Check sheet for the modelled part. Datum: model origin and axes. Units: mm. Face numbers are marked on the shaded views. A direction names the side the tool comes from. Give positions to 0.01 mm unless a question says otherwise; leave off trailing zeros. Order: outer loops, then holes, each group sorted by start corner. A loop starts at its lowest first (then second) coordinate and runs counter-clockwise, first axis right, second up. Notation, with made-up numbers: (47, 78.5) -> (83, 78.5) arc R14 ccw to (83, 87.5) -> close; hole circle Ø8 at (78.5, -37.75). An arc over 180 degrees is marked (long way). Answer in a Markdown table with one row per item. Add a question column.
(1) Set-up check for the marked faces 4, 5 and 6: record each of +Z, -Z, +X, -X, +Y, -Y from which the full face is reachable in a straight line by a thin tool's end or side.
(2) Cross-section at B-B (x = -26). Record the cut outline in (y, z).
(3) Thickness scan on L1, parallel to Z at x = -17.5, y = 36.5; L2, parallel to Y at x = -31, z = 6.5; L3, parallel to Z at x = -26.5, y = 9. Record the ranges inside material, lowest first. Write a range as [from, to].
(4) Go/stop test with flat-tipped pins: pin 1 (6.5 mm diameter, centred on y = 27.5, z = -4, fed in from +X); pin 2 (1 mm diameter, centred on x = -15.5, y = 33, fed in from -Z); pin 3 (2 mm diameter, centred on y = 8.5, z = 23.5, fed in from -X). Record where each tip stops, or that it passes through.
(5) Cross-section at A-A (z = 0). Record the cut outline in (x, y), then the cut area to 3 significant figures.
(6) Release check for a two-part mould opening along Y. For the marked faces 1, 2 and 3 record: released by +Y, released by -Y, zero draft, split by the parting line, or undercut.
(7) Cross-section at D-D (x = 0). Record the cut outline in (y, z).
(8) Cross-section at C-C (y = 26). Record the cut outline in (x, z).
```python
from build123d import *

# Parameters (mm, degrees)
SKETCH1_R           = 41.8
BOSS_EXTRUDE1_DEPTH = 9.5
SKETCH2_W           = 44
SKETCH2_H           = 40.2
BOSS_EXTRUDE2_DEPTH = 28.5
SKETCH3_R           = 4
BOSS_EXTRUDE3_DEPTH = 7.5


with BuildPart() as part:
    # Sketch1 → Boss-Extrude1 (new body)
    with BuildSketch(Plane(origin=(0, 0, 0), x_dir=(1, 0, 0), z_dir=(0, 1, 0))):
        Circle(SKETCH1_R)
    extrude(amount=BOSS_EXTRUDE1_DEPTH)

    # Sketch2 → Boss-Extrude2 (add)
    with BuildSketch(Plane(origin=(0, 9.5, 0), x_dir=(1, 0, 0), z_dir=(0, 1, 0))):
        with Locations((0, -4.7)):
            Rectangle(SKETCH2_W, SKETCH2_H)
    extrude(amount=BOSS_EXTRUDE2_DEPTH)

    # Sketch3 → Boss-Extrude3 (add)
    with BuildSketch(Plane(origin=(22, 0, 0), x_dir=(0, 0, -1), z_dir=(1, 0, 0))):
        with Locations((5.2, 28)):
            Circle(SKETCH3_R)
    boss_extrude3 = extrude(amount=BOSS_EXTRUDE3_DEPTH)

    # Mirror2: Boss-Extrude3 across plane
    add(boss_extrude3.mirror(Plane(origin=(0, 0, 0), x_dir=(0, 0, 1), z_dir=(1, 0, 0))))


solid = part.part
```
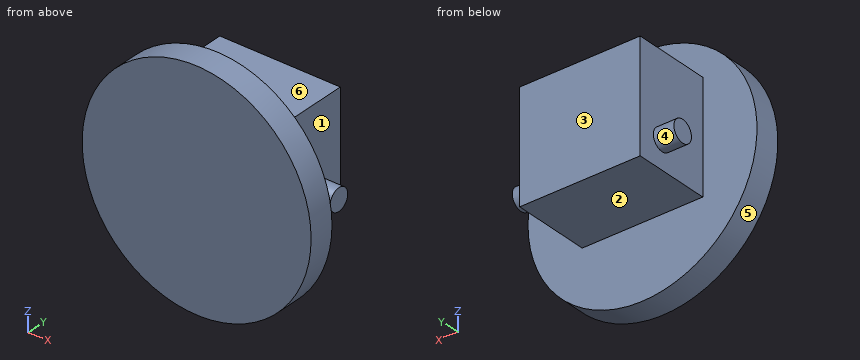
Answer below:
| question | item | result |
|---|---|---|
| 1 | face 4 | -X |
| 1 | face 5 | +Y, -Y |
| 1 | face 6 | +Z, +X, -X, +Y |
| 2 | outline | (0, -32.73) -> (9.5, -32.73) -> (9.5, 32.73) -> (0, 32.73) -> close; circle Ø8 at (28, -5.2) |
| 3 | L1 | z = [-15.4, 24.8] |
| 3 | L2 | y = [0, 9.5] |
| 3 | L3 | z = [-32.33, 32.33] |
| 4 | pin 1 | stops at x = 29.5 |
| 4 | pin 2 | stops at z = -15.4 |
| 4 | pin 3 | stops at x = -35.23 |
| 5 | outline | (-41.8, 0) -> (41.8, 0) -> (41.8, 9.5) -> (22, 9.5) -> (22, 38) -> (-22, 38) -> (-22, 9.5) -> (-41.8, 9.5) -> close |
| 5 | area | 2,050 mm² |
| 6 | face 1 | undercut |
| 6 | face 2 | zero draft |
| 6 | face 3 | released by +Y |
| 7 | outline | (0, -41.8) -> (9.5, -41.8) -> (9.5, -15.4) -> (38, -15.4) -> (38, 24.8) -> (9.5, 24.8) -> (9.5, 41.8) -> (0, 41.8) -> close |
| 8 | outline | (-29.5, -8.66) -> (-22, -8.66) -> (-22, -15.4) -> (22, -15.4) -> (22, -8.66) -> (29.5, -8.66) -> (29.5, -1.74) -> (22, -1.74) -> (22, 24.8) -> (-22, 24.8) -> (-22, -1.74) -> (-29.5, -1.74) -> close |
